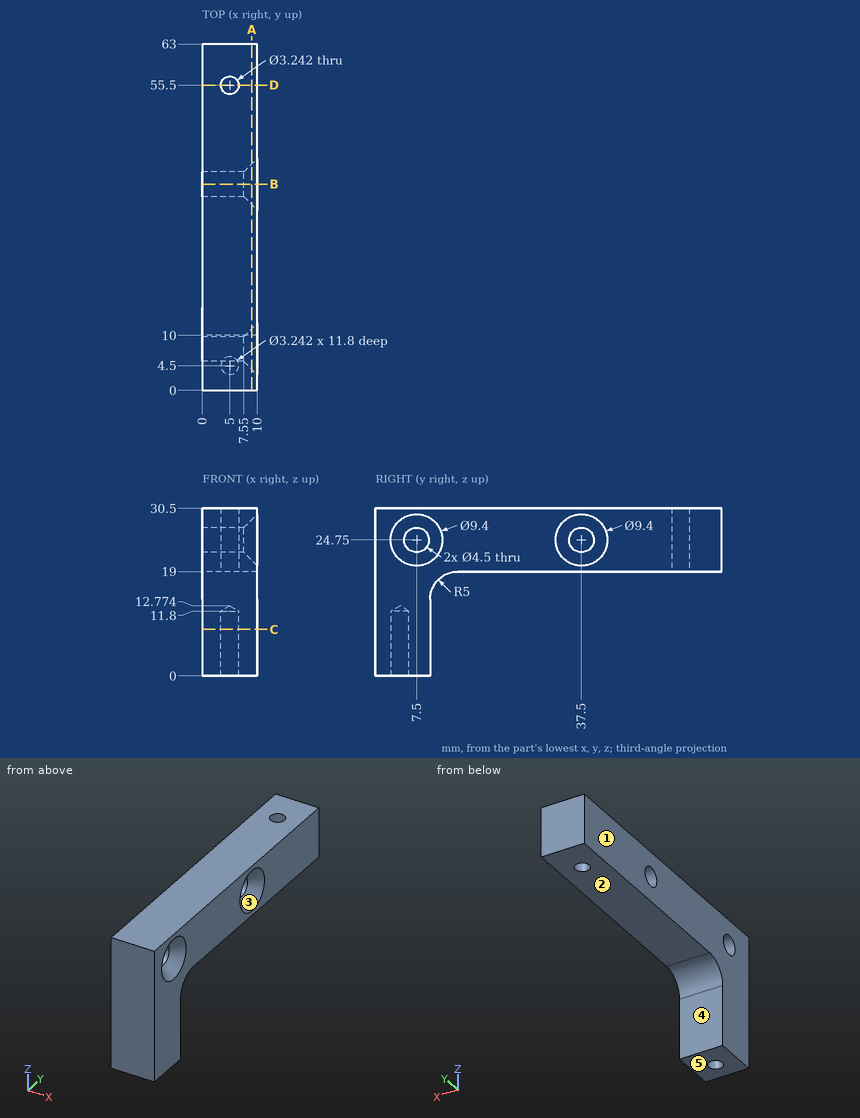
The figure shows three views and two pictorial views of one solid part (mm, origin at its lowest corner). Answer the questions. A direction names the side the tool comes from. Give positions to 0.01 mm unless a question says otherwise; leave off trailing zeros. Loops run counter-clockwise (first coordinate to the right, second up) from the corner with the lowest first, then second, coordinate; pieces in that order, holes last. Notation, with made-up numbers: (1, -25.5) -> (60, -25.5) arc R18 ccw to (60, -16.5) -> close; hole circle Ø7 at (-7.5, 56.5). An arc over 180 degrees is marked (long way). Use a Markdown table: item, result. Add a question column.
1. Section C-C on z = 8.5 is taken. Determine the outline of the cut face in (x, y), and give its area (3 significant figures).
2. Determine the mould class of the marked faces 1, 2 and 3 for opening direction Z: released by +Z, released by -Z, zero draft, split by the parting line, or undercut.
3. Flat-ended cylindrical pins translate along their axes: pin 1 Ø5 at (x, z) = (6, 5.5) entering from +Y; pin 2 Ø1.5 at (y, z) = (34, 26.5) entering from +X; pin 3 Ø5 at (y, z) = (7.5, 24.75) entering from +X. Find the tip coordinate at first contact, or state that the pin passes through.
4. Section B-B on y = 37.5 is taken. Determine the outline of the cut face in (x, z).
5. Find the intervals of material crossed by probe 1 along Y at (x, z) = (1.75, 24.75); probe 2 along Y at (x, z) = (5, 21); probe 3 along Z at (x, y) = (3.75, 37.5), in increasing order.
6. Section A-A on x = 9 is taken. Determine the outline of the cut face in (y, z), and give its area (3 significant figures).
7. Section D-D on y = 55.5 is taken. Determine the outline of the cut face in (x, z), and give its area (3 significant figures).
8. For the marked faces 4 and 5, determine the directions among +Z, -Z, +X, -X, +Y, -Y from which every point of the face is accessible in a straight line to the end or side of a thin tool.
Results below:
| question | item | result |
|---|---|---|
| 1 | outline | (0, 0) -> (10, 0) -> (10, 10) -> (0, 10) -> close; hole circle Ø3.24 at (5, 4.5) |
| 1 | area | 91.7 mm^2 |
| 2 | face 1 | zero draft |
| 2 | face 2 | released by -Z |
| 2 | face 3 | undercut |
| 3 | pin 1 | stops at y = 10 |
| 3 | pin 2 | stops at x = 9.96 |
| 3 | pin 3 | stops at x = 7.8 |
| 4 | outline | (0, 19) -> (10, 19) -> (10, 20.05) -> (7.55, 22.5) -> (0, 22.5) -> close; (0, 27) -> (7.55, 27) -> (10, 29.45) -> (10, 30.5) -> (0, 30.5) -> close |
| 5 | probe 1 | y = 0 to 5.25, 9.75 to 35.25, 39.75 to 63 |
| 5 | probe 2 | y = 0 to 53.88, 57.12 to 63 |
| 5 | probe 3 | z = 19 to 22.5, 27 to 30.5 |
| 6 | outline | (0, 0) -> (10, 0) -> (10, 14) arc R5 cw to (15, 19) -> (63, 19) -> (63, 30.5) -> (0, 30.5) -> close; hole circle Ø7.4 at (7.5, 24.75); hole circle Ø7.4 at (37.5, 24.75) |
| 6 | area | 834 mm^2 |
| 7 | outline | (0, 19) -> (3.38, 19) -> (3.38, 30.5) -> (0, 30.5) -> close; (6.62, 19) -> (10, 19) -> (10, 30.5) -> (6.62, 30.5) -> close |
| 7 | area | 77.7 mm^2 |
| 8 | face 4 | -Z, +X, -X, +Y |
| 8 | face 5 | -Z, +X, -X, +Y, -Y |
